Build history of the part. All positions in model axes, mm. Round coordinates to 2 decimals unless told otherwise and drop trailing zeros. Order: outer loops, then holes, each group sorted by start corner. A loop starts at its lowest first (then second) coordinate and runs counter-clockwise, first axis right, second up. Notation, with made-up numbers: (-38.75, -11) -> (20.25, -11) arc R34 ccw to (20.25, 26) -> close; hole circle Ø7 at (-0.75, -5.5). An arc over 180 degrees is marked (long way). Use a Markdown table: item, result. Add a question column.
Item 1: Slice it at B-B, the plane y = 0.7. State how many separate pieces and enclosed holes the cut face has, plus the area to 3 significant figures.
Item 2: Slice it at A-A, the plane z = 192. Give the cut face in (x, y).
Item 3: Pin check, flat tip, straight feed: pin 1 (1 mm diameter, centred on x = 10, y = 1.5, fed in from +Z). Stop position of the tip, or through.
Item 4: Two-plate mould, pull along Z, no slides. Class faces 1 (the face through (-0.71, 0.99, 214.29)), 2 (the face through (0.297, 0.986, 269.497)), 3 (the face through (-0.297, 0.986, 114.503)): released by +Z, released by -Z, zero draft, split by the parting line, or undercut.
Item 5: Probe L1, parallel to X at y = 1.25, z = 128; L2, parallel to X at y = 1.15, z = 144; L3, parallel to X at y = 0.85, z = 122.34. List the from-to ranges inside material, lowest first.
Autodesk Inventor part; units mm, degrees
ref_plane "YZ Plane" through (0, 0, 0) normal (1, 0, 0) x (0, 1, 0)
ref_plane "XZ Plane" through (0, 0, 0) normal (0, 1, 0) x (-1, 0, 0)
ref_plane "XY Plane" through (0, 0, 0) normal (0, 0, 1) x (1, 0, 0)
sketch "Sketch1" plane through (0, 0, 0) normal (0, 1, 0) x (-1, 0, 0)
  arc A0 (-5.66, 120.49) -> (-5.66, 124.19) centre (-5.66, 122.34) ccw
  arc A1 (-5.66, 124.19) -> (-5.66, 120.49) centre (-5.66, 122.34) ccw
  arc A2 (5.66, 120.49) -> (5.66, 124.19) centre (5.66, 122.34) ccw
  arc A3 (5.66, 124.19) -> (5.66, 120.49) centre (5.66, 122.34) ccw
  arc A4 (0, 134.15) -> (0, 137.85) centre (0, 136) ccw
  arc A5 (0, 137.85) -> (0, 134.15) centre (0, 136) ccw
  arc A6 (-5.66, 131.81) -> (-5.66, 135.51) centre (-5.66, 133.66) ccw
  arc A7 (-5.66, 135.51) -> (-5.66, 131.81) centre (-5.66, 133.66) ccw
  arc A8 (5.66, 131.81) -> (5.66, 135.51) centre (5.66, 133.66) ccw
  arc A9 (5.66, 135.51) -> (5.66, 131.81) centre (5.66, 133.66) ccw
  arc A10 (8, 126.15) -> (8, 129.85) centre (8, 128) ccw
  arc A11 (8, 129.85) -> (8, 126.15) centre (8, 128) ccw
  arc A12 (0, 124) -> (0, 132) centre (0, 128) ccw
  arc A13 (0, 132) -> (0, 124) centre (0, 128) ccw
  arc A14 (-8, 126.15) -> (-8, 129.85) centre (-8, 128) ccw
  arc A15 (-8, 129.85) -> (-8, 126.15) centre (-8, 128) ccw
  arc A16 (0, 118.15) -> (0, 121.85) centre (0, 120) ccw
  arc A17 (0, 121.85) -> (0, 118.15) centre (0, 120) ccw
  arc A18 (-5.66, 195.81) -> (-5.66, 199.51) centre (-5.66, 197.66) ccw
  arc A19 (-5.66, 199.51) -> (-5.66, 195.81) centre (-5.66, 197.66) ccw
  arc A20 (-5.66, 184.49) -> (-5.66, 188.19) centre (-5.66, 186.34) ccw
  arc A21 (-5.66, 188.19) -> (-5.66, 184.49) centre (-5.66, 186.34) ccw
  arc A22 (5.66, 184.49) -> (5.66, 188.19) centre (5.66, 186.34) ccw
  arc A23 (5.66, 188.19) -> (5.66, 184.49) centre (5.66, 186.34) ccw
  arc A24 (5.66, 195.81) -> (5.66, 199.51) centre (5.66, 197.66) ccw
  arc A25 (5.66, 199.51) -> (5.66, 195.81) centre (5.66, 197.66) ccw
  arc A26 (8, 190.15) -> (8, 193.85) centre (8, 192) ccw
  arc A27 (8, 193.85) -> (8, 190.15) centre (8, 192) ccw
  arc A28 (-8, 190.15) -> (-8, 193.85) centre (-8, 192) ccw
  arc A29 (-8, 193.85) -> (-8, 190.15) centre (-8, 192) ccw
  arc A30 (0, 198.15) -> (0, 201.85) centre (0, 200) ccw
  arc A31 (0, 201.85) -> (0, 198.15) centre (0, 200) ccw
  arc A32 (0, 182.15) -> (0, 185.85) centre (0, 184) ccw
  arc A33 (0, 185.85) -> (0, 182.15) centre (0, 184) ccw
  arc A34 (0, 188) -> (0, 196) centre (0, 192) ccw
  arc A35 (0, 196) -> (0, 188) centre (0, 192) ccw
  arc A36 (8, 158.15) -> (8, 161.85) centre (8, 160) ccw
  arc A37 (8, 161.85) -> (8, 158.15) centre (8, 160) ccw
  arc A38 (-8, 158.15) -> (-8, 161.85) centre (-8, 160) ccw
  arc A39 (-8, 161.85) -> (-8, 158.15) centre (-8, 160) ccw
  arc A40 (0, 166.15) -> (0, 169.85) centre (0, 168) ccw
  arc A41 (0, 169.85) -> (0, 166.15) centre (0, 168) ccw
  arc A42 (0, 150.15) -> (0, 153.85) centre (0, 152) ccw
  arc A43 (0, 153.85) -> (0, 150.15) centre (0, 152) ccw
  arc A44 (0, 156) -> (0, 164) centre (0, 160) ccw
  arc A45 (0, 164) -> (0, 156) centre (0, 160) ccw
  arc A46 (-5.66, 248.49) -> (-5.66, 252.19) centre (-5.66, 250.34) ccw
  arc A47 (-5.66, 252.19) -> (-5.66, 248.49) centre (-5.66, 250.34) ccw
  arc A48 (5.66, 248.49) -> (5.66, 252.19) centre (5.66, 250.34) ccw
  arc A49 (5.66, 252.19) -> (5.66, 248.49) centre (5.66, 250.34) ccw
  arc A50 (0, 262.15) -> (0, 265.85) centre (0, 264) ccw
  arc A51 (0, 265.85) -> (0, 262.15) centre (0, 264) ccw
  arc A52 (-5.66, 259.81) -> (-5.66, 263.51) centre (-5.66, 261.66) ccw
  arc A53 (-5.66, 263.51) -> (-5.66, 259.81) centre (-5.66, 261.66) ccw
  arc A54 (5.66, 259.81) -> (5.66, 263.51) centre (5.66, 261.66) ccw
  arc A55 (5.66, 263.51) -> (5.66, 259.81) centre (5.66, 261.66) ccw
  arc A56 (8, 254.15) -> (8, 257.85) centre (8, 256) ccw
  arc A57 (8, 257.85) -> (8, 254.15) centre (8, 256) ccw
  arc A58 (0, 252) -> (0, 260) centre (0, 256) ccw
  arc A59 (0, 260) -> (0, 252) centre (0, 256) ccw
  arc A60 (8, 222.15) -> (8, 225.85) centre (8, 224) ccw
  arc A61 (8, 225.85) -> (8, 222.15) centre (8, 224) ccw
  arc A62 (-8, 222.15) -> (-8, 225.85) centre (-8, 224) ccw
  arc A63 (-8, 225.85) -> (-8, 222.15) centre (-8, 224) ccw
  arc A64 (0, 230.15) -> (0, 233.85) centre (0, 232) ccw
  arc A65 (0, 233.85) -> (0, 230.15) centre (0, 232) ccw
  arc A66 (0, 214.15) -> (0, 217.85) centre (0, 216) ccw
  arc A67 (0, 217.85) -> (0, 214.15) centre (0, 216) ccw
  arc A68 (0, 220) -> (0, 228) centre (0, 224) ccw
  arc A69 (0, 228) -> (0, 220) centre (0, 224) ccw
  arc A70 (0, 140) -> (0, 148) centre (0, 144) ccw
  arc A71 (0, 148) -> (0, 140) centre (0, 144) ccw
  arc A72 (0.1754, 172) -> (0.1754, 180) centre (0.1754, 176) ccw
  arc A73 (0.1754, 180) -> (0.1754, 172) centre (0.1754, 176) ccw
  arc A74 (0, 204) -> (0, 212) centre (0, 208) ccw
  arc A75 (0, 212) -> (0, 204) centre (0, 208) ccw
  arc A76 (0, 236) -> (0, 244) centre (0, 240) ccw
  arc A77 (0, 244) -> (0, 236) centre (0, 240) ccw
  arc A78 (-8, 254.15) -> (-8, 257.85) centre (-8, 256) ccw
  arc A79 (-8, 257.85) -> (-8, 254.15) centre (-8, 256) ccw
  arc A80 (0, 246.15) -> (0, 249.85) centre (0, 248) ccw
  arc A81 (0, 249.85) -> (0, 246.15) centre (0, 248) ccw
  arc A82 (13.5, 256) -> (0, 269.5) centre (0, 256) ccw
  arc A83 (0, 269.5) -> (-13.5, 256) centre (0, 256) ccw
  line L0 (-13.5, 256) -> (-13.5, 128)
  line L1 (13.5, 128) -> (13.5, 256)
  arc A84 (2.852, 141.1953) -> (-2.852, 141.1953) centre (0, 128) ccw
  arc A85 (-13.5, 128) -> (13.5, 128) centre (0, 128) ccw
  point P0 (0, 0)
  point P1 (0, 128)
extrude "Extrusion1" add sketch "Sketch1" along normal blind 2
properties part number "Tetrix Flat bar 160 mm"
Check sheet entries:
| question | item | result |
|---|---|---|
| 1 | separate pieces | 1 |
| 1 | enclosed holes | 41 |
| 1 | area | 3,230 mm2 |
| 2 | outline | (-13.5, 0) -> (-9.85, 0) -> (-9.85, 2) -> (-13.5, 2) -> close; (-6.15, 0) -> (-4, 0) -> (-4, 2) -> (-6.15, 2) -> close; (4, 0) -> (6.15, 0) -> (6.15, 2) -> (4, 2) -> close; (9.85, 0) -> (13.5, 0) -> (13.5, 2) -> (9.85, 2) -> close |
| 3 | pin 1 | z = 265.59 |
| 4 | face 1 | undercut |
| 4 | face 2 | released by +Z |
| 4 | face 3 | released by -Z |
| 5 | L1 | -13.5 to -9.85, -6.15 to -4, 4 to 6.15, 9.85 to 13.5 |
| 5 | L2 | -13.5 to -4, 4 to 13.5 |
| 5 | L3 | -12.26 to -7.51, -3.81 to 3.81, 7.51 to 12.26 |
